from build123d import *

# Parameters (mm, degrees)
SKETCH1_R           = 1.905
SKETCH1_R_2         = 1.3890625
BOSS_EXTRUDE1_DEPTH = 6.35


with BuildPart() as part:
    # Sketch1 → Boss-Extrude1 (new body)
    with BuildSketch(Plane.XY):
        with BuildLine():
            Line((12.7, 0), (-12.7, 0))
            Line((-12.7, 0), (-12.7, -39.593860647))
            Line((-12.7, -39.593860647), (-23.8125, -39.593860647))
            Line((-23.8125, -39.593860647), (-23.8125, 1.27))
            add(Edge.make_bspline(
                [(-23.8125, 1.27), (-23.8125, 28.224807165), (-50.502986928, 35.738173469)],
                knots=[0, 0, 0, 1.28831511, 1.28831511, 1.28831511], degree=2, weights=[1, 0.79960596, 1]))
            ThreePointArc((-50.502986928, 35.738173469), (-53.573053894, 42.237434983), (-46.71026588, 44.374688379))
            ThreePointArc((-46.71026588, 44.374688379), (0, 31.115), (46.71026588, 44.374688379))
            ThreePointArc((46.71026588, 44.374688379), (53.573053894, 42.237434983), (50.502986928, 35.738173469))
            add(Edge.make_bspline(
                [(50.502986928, 35.738173469), (23.8125, 28.224807165), (23.8125, 1.27)],
                knots=[1.853277544, 1.853277544, 1.853277544, 3.141592654, 3.141592654, 3.141592654], degree=2, weights=[1, 0.79960596, 1]))
            Line((23.8125, 1.27), (23.8125, -5.08))
            Line((23.8125, -5.08), (23.8125, -39.593860647))
            Line((23.8125, -39.593860647), (12.7, -39.593860647))
            Line((12.7, -39.593860647), (12.7, 0))
        make_face()
        with Locations((-19.05, -15.875)):
            Circle(SKETCH1_R, mode=Mode.SUBTRACT)
        with Locations(Location((19.05, -15.875, 0), (0, 0, 180))):
            Circle(SKETCH1_R, mode=Mode.SUBTRACT)
        with Locations((-49.2125, 40.3225)):
            Circle(SKETCH1_R_2, mode=Mode.SUBTRACT)
        with Locations((-19.05, -34.925)):
            Circle(SKETCH1_R, mode=Mode.SUBTRACT)
        with Locations(Location((19.05, -34.925, 0), (0, 0, 180))):
            Circle(SKETCH1_R, mode=Mode.SUBTRACT)
        with Locations(Location((49.2125, 40.3225, 0), (0, 0, 180))):
            Circle(SKETCH1_R_2, mode=Mode.SUBTRACT)
    extrude(amount=BOSS_EXTRUDE1_DEPTH)


solid = part.part
Verification items for the finished model (mm, model axes). A direction names the side the tool comes from. Give positions to 0.01 mm unless a question says otherwise; leave off trailing zeros. Loops run counter-clockwise (first coordinate to the right, second up) from the corner with the lowest first, then second, coordinate; pieces in that order, holes last. Notation, with made-up numbers: (-24, 3) - (28, 3) arc R33 ccw to (28, 40) - close; hole circle Ø5 at (-2.75, 9). An arc over 180 degrees is marked (long way). Write each question's results on one line, items separated by ' | '.
1) Sectioned sample at C-C on z = 3. Count the separate pieces of the cut face and the enclosed holes in it, plus the area to 3 significant figures.
Solution:
separate pieces: 1 | enclosed holes: 6 | area: 3,090 mm2
2) Tool access check on faces 1 (the flat face through (-12.7, -20, 3)), 2 (the flat face through (23.812, -19, 3)), 3 (the cylindrical face through (50.236, 39.384, 3.131)). Record the directions out of +Z, -Z, +X, -X, +Y, -Y that give a thin tool (end or side, any length) a straight path to the whole face; none if there is none.
Solution:
face 1: +Z, -Z, -Y | face 2: +Z, -Z, +X, -Y | face 3: +Z, -Z
3) Depth check by flat-ended pin: P1, Ø1, axis at x = 22, y = -25, coming from the -Z side; P2, Ø3, axis at y = -24.5, z = 5, coming from the +X side; P3, Ø2.5, axis at x = -49.21, y = 40.32, coming from the +Z side; P4, Ø3, axis at y = -22.5, z = 2.5, coming from the -X side. Enter the tip coordinate at first touch or a pass-through.
Solution:
P1: z = 0 | P2: x = 23.81 | P3: through | P4: x = -23.81
4) Material ranges on L1, parallel to Y at x = -19, z = 4.5; L2, parallel to X at y = -27, z = 4.25; L3, parallel to Y at x = -18.5, z = 6.25, recorded low to high. Write a range as from..to.
Solution:
L1: -39.59..-36.83, -33.02..-17.78, -13.97..33.17 | L2: -23.81..-12.7, 12.7..23.81 | L3: -39.59..-36.75, -33.1..-17.7, -14.05..33.06
5) Mould release check, pull along X, two halves, no side actions. Record for faces 4 (the flat face through (-23.812, -19, 3)), 5 (the flat face through (12.7, -20, 3)), 6 (the flat face through (0, 9, 0)): pulls with the +X half, pulls with the -X half, needs draft (parallel to the pull), parting line crosses it, or undercut.
Solution:
face 4: pulls with the -X half | face 5: undercut | face 6: needs draft
6) Sectioned sample at B-B on x = 19.05. Record the boundary of the cut face in (y, z).
Solution:
outline: (-39.59, 0) - (-36.83, 0) - (-36.83, 6.35) - (-39.59, 6.35) - close; (-33.02, 0) - (-17.78, 0) - (-17.78, 6.35) - (-33.02, 6.35) - close; (-13.97, 0) - (33.18, 0) - (33.18, 6.35) - (-13.97, 6.35) - close
7) Sectioned sample at D-D on x = -14. Record the boundary of the cut face in (y, z), plus the area to 3 significant figures.
Solution:
outline: (-39.59, 0) - (32.22, 0) - (32.22, 6.35) - (-39.59, 6.35) - close | area: 456 mm2
8) Sectioned sample at A-A on y = -26.5. Record the boundary of the cut face in (x, z).
Solution:
outline: (-23.81, 0) - (-12.7, 0) - (-12.7, 6.35) - (-23.81, 6.35) - close; (12.7, 0) - (23.81, 0) - (23.81, 6.35) - (12.7, 6.35) - close
